Geometry check sheet. Reference: drawing and pictorial views, mm from the part's lowest x, y, z. Round coordinates to 2 decimals unless told otherwise and drop trailing zeros. Order: outer loops, then holes, each group sorted by start corner. A loop starts at its lowest first (then second) coordinate and runs counter-clockwise, first axis right, second up. Notation, with made-up numbers: (63.5, 27) -> (116.5, 27) arc R18 cw to (116.5, 52) -> close; hole circle Ø10 at (77.25, 50.25). An arc over 180 degrees is marked (long way). Return JSON: item names as keys, results as strings. Group by question number.
1) Draft check along Z on the marked faces 1, 2, 3 and 4. Enter one of: pulls with the +Z half, pulls with the -Z half, needs draft (parallel to the pull), parting line crosses it, or undercut.
2) Scan lines: L1, parallel to X at y = 1.35, z = 16; L2, parallel to Z at x = 9, y = 8.5. Record each from-to range of solid material in increasing order.
3) Depth check by flat-ended pin: pin 1 (4 mm diameter, centred on y = 4.5, z = 15, fed in from -X); pin 2 (1.7 mm diameter, centred on x = 20.5, z = 16.5, fed in from +Y); pin 3 (3 mm diameter, centred on y = 4.5, z = 9.5, fed in from +X); pin 4 (1.8 mm diameter, centred on x = 32.5, y = 1, fed in from +Z). Enter the tip coordinate at first touch or a pass-through.
4) Section check A-A on x = 37. Enter the section's corners in (y, z).
5) Section check D-D on z = 12. Enter the section's corners in (x, y).
6) Section check C-C on y = 11. Enter the section's corners in (x, z).
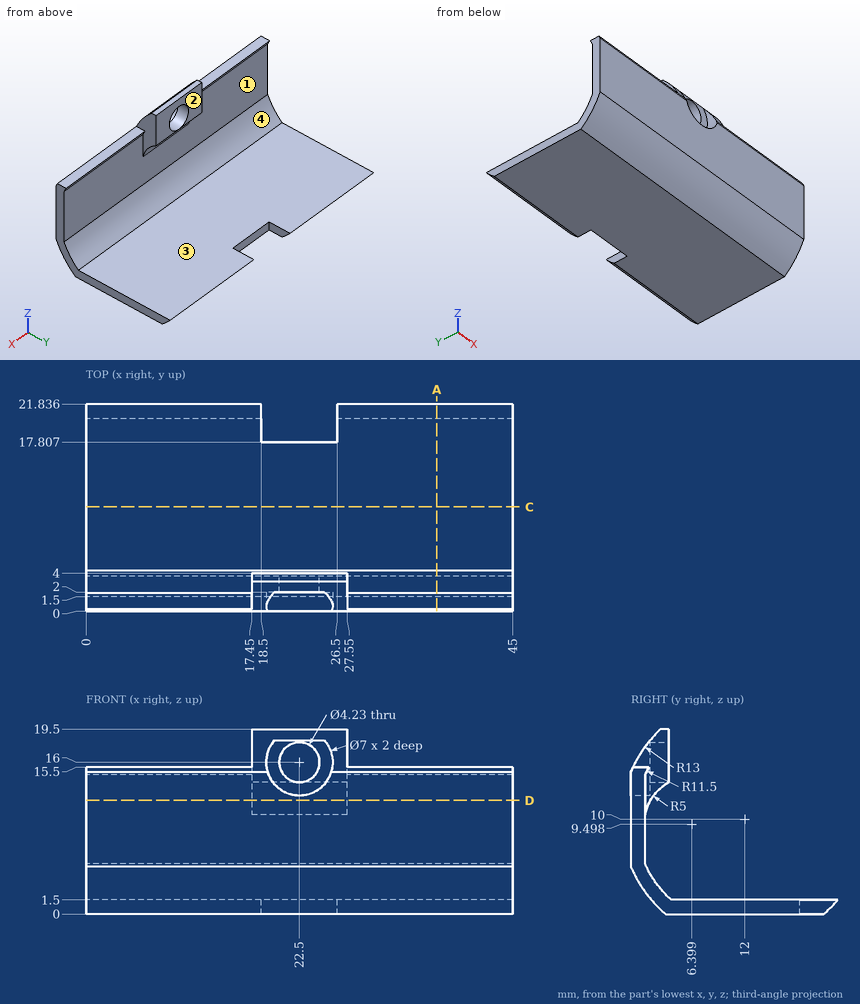
Check result:
{
 "1": {"face 1": "undercut", "face 2": "needs draft", "face 3": "pulls with the +Z half", "face 4": "undercut"},
 "2": {"L1": "17.45 to 19, 26 to 27.55", "L2": "0 to 1.5"},
 "3": {"pin 1": "x = 17.45", "pin 2": "y = 4", "pin 3": "through", "pin 4": "z = 15.5"},
 "4": {"outline": "(0, 5) arc R13 ccw to (3.69, 0) -> (20.31, 0) arc R13 ccw to (21.84, 1.5) -> (4.25, 1.5) arc R11.5 cw to (1.5, 5.31) -> (1.5, 14.69) arc R11.5 cw to (1.9, 15.5) -> (0.22, 15.5) arc R13 ccw to (0, 15) -> close"},
 "5": {"outline": "(0, 0) -> (45, 0) -> (45, 1.5) -> (27.55, 1.5) -> (27.55, 2.07) -> (17.45, 2.07) -> (17.45, 1.5) -> (0, 1.5) -> close"},
 "6": {"outline": "(0, 0) -> (45, 0) -> (45, 1.5) -> (0, 1.5) -> close"}
}
